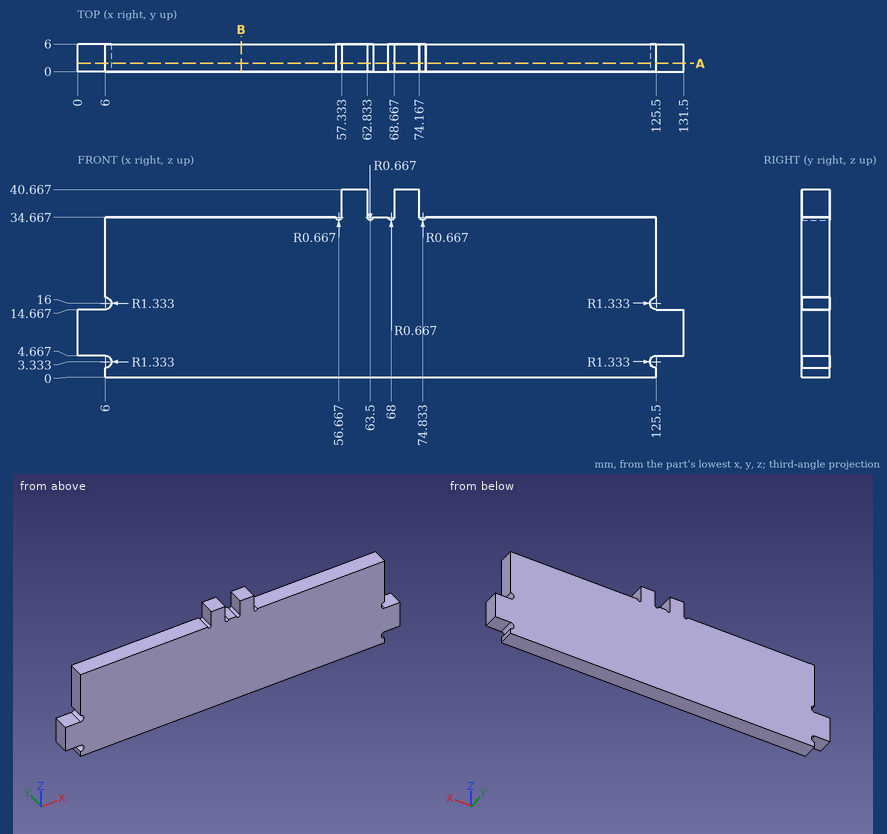
Part print with two shaded views. Sizes in mm from the minimum x, y, z corner. Coordinates: 2 decimals unless noted, no trailing zeros. Loops run counter-clockwise (first coordinate to the right, second up) from the corner with the lowest first, then second, coordinate; pieces in that order, holes last. Notation, with made-up numbers: (79, -21.75) - (133, -21.75) arc R36 ccw to (133, 13.25) - close; hole circle Ø9 at (46.25, -31). An arc over 180 degrees is marked (long way). Write each question's results on one line, items separated by ' | '. Start each with the question number.
Q1. Slice it at B-B on x = 35.5. Give the cut face in (y, z), and give its area (3 significant figures).
Q2. Probe line 1 along X through (y, z) = (1.85, 34.5) (1 decimal); line 2 along X through (y, z) = (4, 38.5); line 3 along Z through (x, y) = (113.5, 3.9). List the from-to ranges inside material, lowest first.
Q3. Drop flat-ended pins along their axis: pin 1 Ø2 at (y, z) = (2, 1.5) entering from -X; pin 2 Ø1.8 at (x, y) = (127.5, 3) entering from -Z; pin 3 Ø1.5 at (x, y) = (84.5, 3.5) entering from +Z. Give the stop position or say it passes through.
Q4. Slice it at A-A on y = 1.8. Give the cut face in (x, z).
Answer:
1) outline: (0, 0) - (6, 0) - (6, 34.67) - (0, 34.67) - close | area: 208 mm2
2) line 1: x = 6 to 56, 57.3 to 62.9, 64.1 to 67.4, 68.6 to 74.2, 75.5 to 125.5 | line 2: x = 57.33 to 62.83, 68.67 to 74.17 | line 3: z = 0 to 34.67
3) pin 1: stops at x = 6 | pin 2: stops at z = 4.67 | pin 3: stops at z = 34.67
4) outline: (0, 4.67) - (6, 4.67) arc R1.33 cw to (6, 2) - (6, 0) - (125.5, 0) - (125.5, 2) arc R1.33 cw to (125.5, 4.67) - (131.5, 4.67) - (131.5, 14.67) - (125.5, 14.67) arc R1.33 cw to (125.5, 17.33) - (125.5, 34.67) - (75.5, 34.67) arc R0.67 cw to (74.17, 34.67) - (74.17, 40.67) - (68.67, 40.67) - (68.67, 34.67) arc R0.67 cw to (67.33, 34.67) - (64.17, 34.67) arc R0.67 cw to (62.83, 34.67) - (62.83, 40.67) - (57.33, 40.67) - (57.33, 34.67) arc R0.67 cw to (56, 34.67) - (6, 34.67) - (6, 17.33) arc R1.33 cw to (6, 14.67) - (0, 14.67) - close
